Design review of the part shown in the three views and the two pictorial views. Dimensions are in mm from the part's minimum x, y and z. A direction names the side the tool comes from. Coordinates: 2 decimals unless noted, no trailing zeros. Loops run counter-clockwise (first coordinate to the right, second up) from the corner with the lowest first, then second, coordinate; pieces in that order, holes last. Notation, with made-up numbers: (0, 57.25) -> (19, 57.25) arc R23 cw to (19, 76.25) -> close; hole circle Ø11 at (22.25, 37). An arc over 180 degrees is marked (long way). One line per item, written item: value.
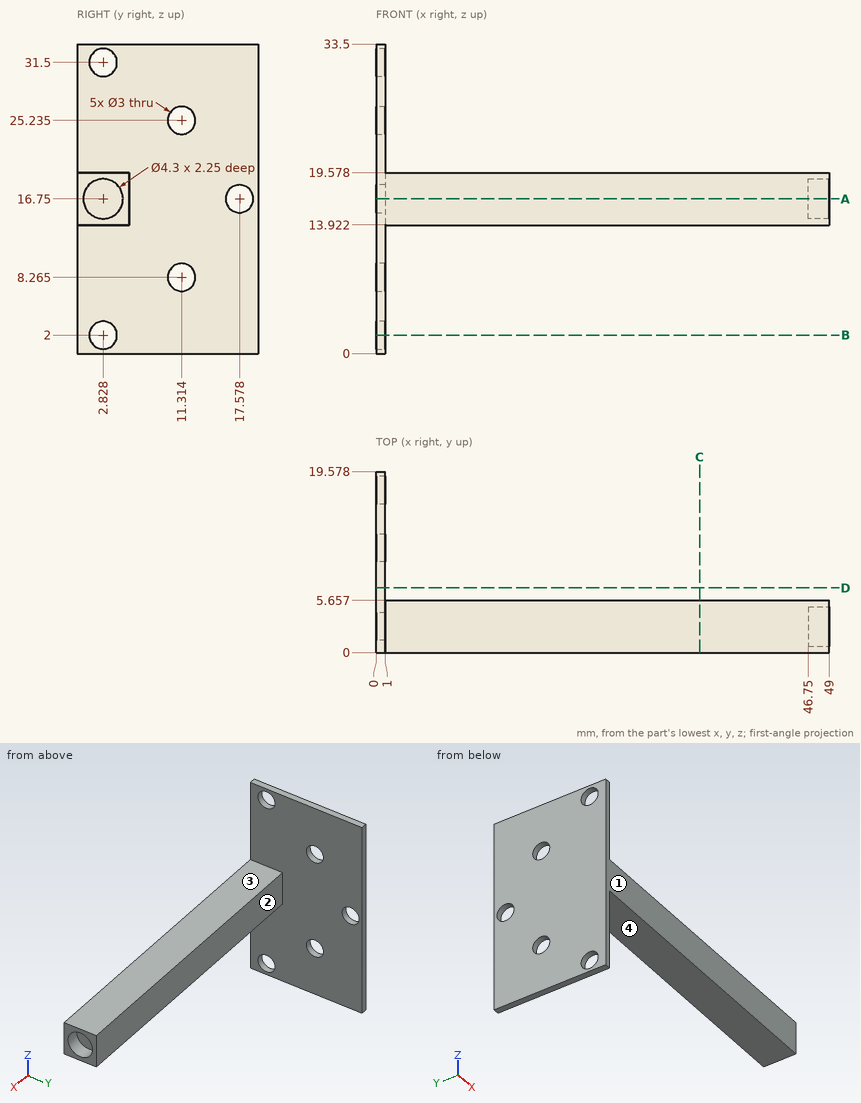
1. Take a section at C-C, the plane x = 35. Give the boundary of the cut face in (y, z).
Return value:
outline: (0, 13.92) -> (5.66, 13.92) -> (5.66, 19.58) -> (0, 19.58) -> close
2. Take a section at A-A, the plane z = 16.75. Give the boundary of the cut face in (x, y).
Return value:
outline: (0, 0) -> (49, 0) -> (49, 0.68) -> (46.75, 0.68) -> (46.75, 4.98) -> (49, 4.98) -> (49, 5.66) -> (1, 5.66) -> (1, 16.08) -> (0, 16.08) -> close; (0, 19.08) -> (1, 19.08) -> (1, 19.58) -> (0, 19.58) -> close
3. Take a section at B-B, the plane z = 2. Give the boundary of the cut face in (x, y).
Return value:
outline: (0, 0) -> (1, 0) -> (1, 1.33) -> (0, 1.33) -> close; (0, 4.33) -> (1, 4.33) -> (1, 19.58) -> (0, 19.58) -> close
4. To check wall thickness, follow probe 1 along Y at (x, z) = (47.4, 16.75); probe 2 along X at (y, z) = (6.5, 31.5); probe 3 along Z at (x, y) = (33, 1). State the ranges of each line that lie inside material, in increasing order. Write a range as from..to.
Return value:
probe 1: y = 0..0.68, 4.98..5.66
probe 2: x = 0..1
probe 3: z = 13.92..19.58
5. For the marked faces 1, 2, 3 and 4, list the 3-axis set-ups (+Z, -Z, +X, -X, +Y, -Y) from which the entire face can be reached by the end or side of a thin tool; tool diameter is ignored.
Return value:
face 1: +Z, -Z, +X, -X, -Y
face 2: +Z, -Z, +X, +Y
face 3: +Z, +X, +Y, -Y
face 4: -Z, +X, +Y, -Y
6. Insertion check: pin 1 Ø5 at (y, z) = (13.5, 26) entering from +X; pin 2 Ø8 at (x, y) = (6.5, 8.5) entering from -Z; pin 3 Ø4.5 at (x, y) = (19.5, 3.5) entering from +Z; pin 4 Ø4.5 at (y, z) = (3, 16.5) entering from +X. Each pin has a flat end and moves straight along its axis. Give the tip position at first contact, or say it passes through.
Return value:
pin 1: stops at x = 1
pin 2: stops at z = 13.92
pin 3: stops at z = 19.58
pin 4: stops at x = 49
7. Take a section at D-D, the plane y = 7. Give the boundary of the cut face in (x, z).
Return value:
outline: (0, 0) -> (1, 0) -> (1, 33.5) -> (0, 33.5) -> close
